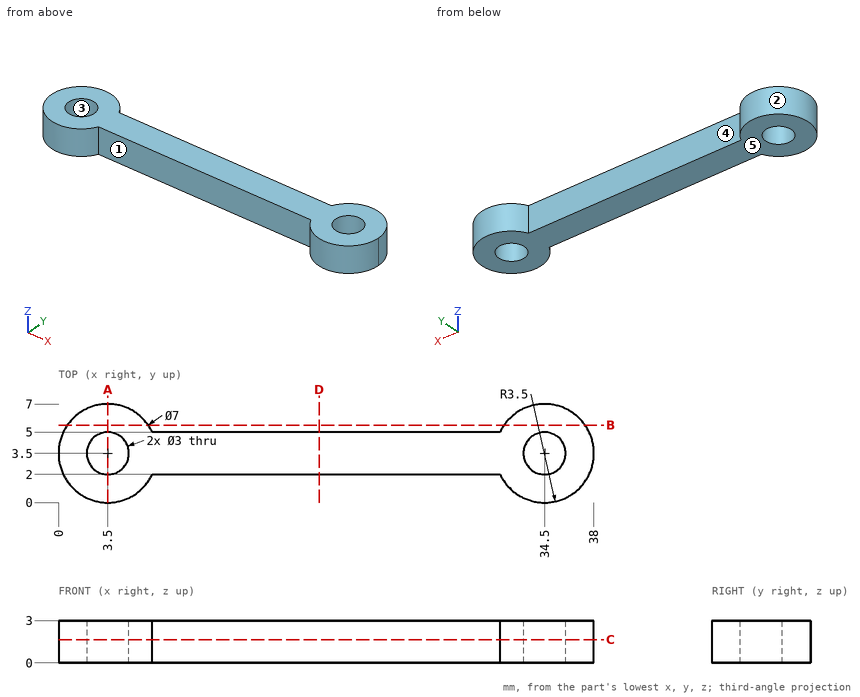
The drawing under review shows one solid part. Ordinate dimensions are in mm from its lowest x, y, z. A direction names the side the tool comes from. Coordinates: 2 decimals unless noted, no trailing zeros. Order: outer loops, then holes, each group sorted by start corner. A loop starts at its lowest first (then second) coordinate and runs counter-clockwise, first axis right, second up. Notation, with made-up numbers: (-31, 25) -> (7, 25) arc R23 cw to (7, 45) -> close; hole circle Ø6 at (84.25, 81). An arc over 180 degrees is marked (long way). One line per item, written item: value.
1) To check wall thickness, follow probe 1 along Y at (x, z) = (34.5, 2.25); probe 2 along Y at (x, z) = (11.5, 2.3); probe 3 along Y at (x, z) = (2.5, 0.4). State the ranges of each line that lie inside material, in increasing order. Write a range as [from, to].
Output values:
probe 1: y = [0, 2], [5, 7]
probe 2: y = [2, 5]
probe 3: y = [0.15, 2.38], [4.62, 6.85]
2) We need section A-A, the plane x = 3.5. Give the boundary of the cut face in (y, z), then the cut area to 3 significant figures.
Output values:
outline: (0, 0) -> (2, 0) -> (2, 3) -> (0, 3) -> close; (5, 0) -> (7, 0) -> (7, 3) -> (5, 3) -> close
area: 12.0 mm2
3) We need section D-D, the plane x = 18.5. Give the boundary of the cut face in (y, z).
Output values:
outline: (2, 0) -> (5, 0) -> (5, 3) -> (2, 3) -> close
4) We need section B-B, the plane y = 5.5. Give the boundary of the cut face in (x, z), then the cut area to 3 significant figures.
Output values:
outline: (0.63, 0) -> (6.37, 0) -> (6.37, 3) -> (0.63, 3) -> close; (31.63, 0) -> (37.37, 0) -> (37.37, 3) -> (31.63, 3) -> close
area: 34.5 mm2
5) Machinability: for the marked faces 1 and 2, which of the approach directions +Z, -Z, +X, -X, +Y, -Y give a long, thin tool a straight path to every point of the face, cutting with its end or side? Answer none if there is none.
Output values:
face 1: +Z, -Z, -Y
face 2: +Z, -Z
6) Clearance check with flat-ended pins moving along their axes: P1, Ø1.5, axis at x = 19.5, z = 1, coming from the -Y side; P2, Ø1, axis at y = 4.5, z = 1, coming from the +X side. State where each tip first meets the part, or that it passes through.
Output values:
P1: stops at y = 2
P2: stops at x = 37.96
7) Draft analysis for pull direction Y (two halves, no side actions). For the marked faces 3, 4 and 5, state which applies: +Y half, -Y half, draft (parallel to the pull), parting line (faces both ways), or undercut.
Output values:
face 3: undercut
face 4: +Y half
face 5: draft
8) We need section C-C, the plane z = 1.65. Give the boundary of the cut face in (x, y), then the cut area to 3 significant figures.
Output values:
outline: (6.66, 2) -> (31.34, 2) arc R3.5 ccw (long way) to (31.34, 5) -> (6.66, 5) arc R3.5 ccw (long way) to start; hole circle Ø3 at (3.5, 3.5); hole circle Ø3 at (34.5, 3.5)
area: 135 mm2
